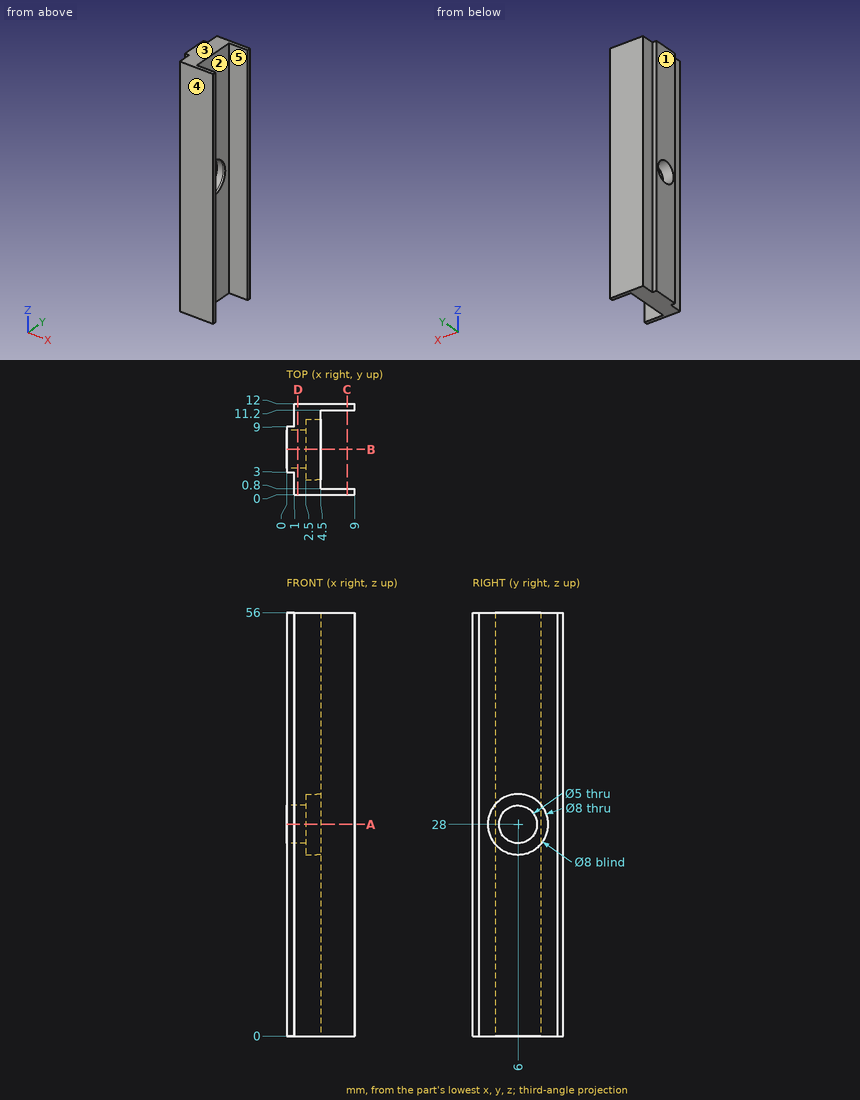
Here's the drawing with two shaded views (mm, measured from the low corner). I have some questions. A direction names the side the tool comes from. Give positions to 0.01 mm unless a question says otherwise; leave off trailing zeros. Loops run counter-clockwise (first coordinate to the right, second up) from the corner with the lowest first, then second, coordinate; pieces in that order, holes last. Notation, with made-up numbers: (-25.75, 31.5) - (-6.75, 31.5) arc R14 cw to (-6.75, 58.5) - close; hole circle Ø6 at (20, 34.5). An arc over 180 degrees is marked (long way). One line per item, written item: value.
(1) If we section it at C-C, the plane x = 8: List the corners of the cut face in (y, z) for me.
Verdict:
outline: (0, 0) - (0.8, 0) - (0.8, 56) - (0, 56) - close; (11.2, 0) - (12, 0) - (12, 56) - (11.2, 56) - close
(2) I'm going to push flat-ended pins straight in: pin 1 (2.5 mm diameter, centred on y = 1, z = 26.5, fed in from -X); pin 2 (0.5 mm diameter, centred on x = 0.5, z = 18, fed in from +Y); pin 3 (4 mm diameter, centred on y = 5.5, z = 27.5, fed in from +X). Where does each tip first touch, or does it pass through?
Verdict:
pin 1: x = 1
pin 2: y = 9
pin 3: x = 2.5
(3) If we section it at A-A, the plane z = 28: List the corners of the cut face in (x, y) for me, plus the area to 3 significant figures.
Verdict:
outline: (0, 3) - (1, 3) - (1, 0) - (9, 0) - (9, 0.8) - (4.5, 0.8) - (4.5, 2) - (2.5, 2) - (2.5, 3.5) - (0, 3.5) - close; (0, 8.5) - (2.5, 8.5) - (2.5, 10) - (4.5, 10) - (4.5, 11.2) - (9, 11.2) - (9, 12) - (1, 12) - (1, 9) - (0, 9) - close
area: 26.7 mm^2
(4) If we section it at B-B, the plane y = 6: List the corners of the cut face in (x, z) for me, plus the area to 4 significant figures.
Verdict:
outline: (0, 0) - (4.5, 0) - (4.5, 24) - (2.5, 24) - (2.5, 25.5) - (0, 25.5) - close; (0, 30.5) - (2.5, 30.5) - (2.5, 32) - (4.5, 32) - (4.5, 56) - (0, 56) - close
area: 223.5 mm^2
(5) On a 3-axis mill with a long thin cutter (end or side, diameter ignored), from which of +Z, -Z, +X, -X, +Y, -Y can I reach the whole of each face in a straight line? I mean the marked faces 1 and 2. Say none if no direction works.
Verdict:
face 1: +Z, -Z, -X, +Y, -Y
face 2: +Z, -Z, +X
(6) If we mould it in two halves opening along Y, with no side actions, what happens to the marked faces 3, 4 and 5? For each: released by +Y, released by -Y, zero draft, split by the parting line, or undercut.
Verdict:
face 3: zero draft
face 4: released by -Y
face 5: undercut
(7) If we section it at D-D, the plane x = 1.5: List the corners of the cut face in (y, z) for me.
Verdict:
outline: (0, 0) - (12, 0) - (12, 56) - (0, 56) - close; hole circle Ø5 at (6, 28)
(8) I need wall thicknesses on line 1 along Z through (x, y) = (3.2, 6); line 2 along Y through (x, z) = (0.5, 6); line 3 along X through (y, z) = (3.75, 45.5). Which ranges of each line are inside material? Lowest first, please.
Verdict:
line 1: 0 to 24, 32 to 56
line 2: 3 to 9
line 3: 0 to 4.5
